Part model, mm, in its own coordinate system. Round coordinates to 2 decimals unless told otherwise and drop trailing zeros. Order: outer loops, then holes, each group sorted by start corner. A loop starts at its lowest first (then second) coordinate and runs counter-clockwise, first axis right, second up. Notation, with made-up numbers: (-12, -31.75) - (24, -31.75) arc R32 ccw to (24, 2.25) - close; hole circle Ø7 at (74, 56.5). An arc over 180 degrees is marked (long way). Answer as a JSON object with one key per item and string values.
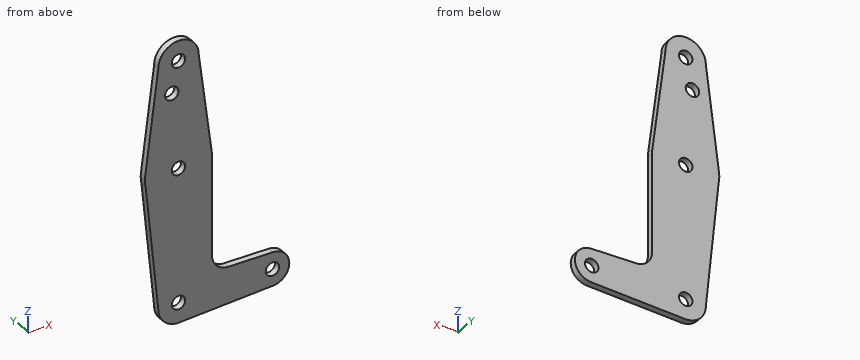
```python
from build123d import *

# Parameters (mm, degrees)
F0_R     = 3.175
F1_DEPTH = 3.048


with BuildPart() as f1:
    # F0 (on Front) → F1 (new body)
    with BuildSketch(Plane.XZ):
        with BuildLine():
            ThreePointArc((3.175, 0), (-2.2450640303, -2.2450640303), (0, 3.175))
            Line((0, 3.175), (0, 9.525))
            ThreePointArc((0, 9.525), (-6.7351920908, 6.7351920908), (-9.525, 0))
            ThreePointArc((-9.525, 0), (-6.7351920908, -6.7351920908), (0, -9.525))
            Line((0, -9.525), (0.6773435479, -9.500885786))
            ThreePointArc((0.6773435479, -9.500885786), (6.9705567315, -6.4912990883), (9.525, 0))
            Line((9.525, 0), (3.175, 0))
        make_face()
        with BuildLine():
            ThreePointArc((-9.525, 0), (-6.7351920908, 6.7351920908), (0, 9.525))
            Line((0, 9.525), (0, 47.625))
            ThreePointArc((0, 47.625), (-10.0526499203, 51.2134278751), (-15.5606435644, 60.3564356436))
            Line((-15.5606435644, 60.3564356436), (-9.525, 0))
        make_face()
        with BuildLine():
            Line((0, 47.625), (0, 9.525))
            ThreePointArc((0, 9.525), (6.7351920908, 6.7351920908), (9.525, 0))
            Line((9.525, 0), (36.5125, 0))
            ThreePointArc((36.5125, 0), (38.9239306999, 5.6979350945), (44.6930264481, 7.9337786959))
            Line((44.6930264481, 7.9337786959), (23.5817847096, 8.5804554297))
            ThreePointArc((23.5817847096, 8.5804554297), (18.1181482094, 10.9920171606), (15.875, 16.5269281715))
            Line((15.875, 16.5269281715), (15.875, 63.5))
            ThreePointArc((15.875, 63.5), (11.2253201513, 52.2746798487), (0, 47.625))
        make_face()
        with BuildLine():
            Line((36.5125, 0), (9.525, 0))
            ThreePointArc((9.525, 0), (6.9705567315, -6.4912990883), (0.6773435479, -9.500885786))
            Line((0.6773435479, -9.500885786), (44.7324052746, -7.9324746146))
            ThreePointArc((44.7324052746, -7.9324746146), (38.9380895153, -5.7116327839), (36.5125, 0))
        make_face()
        with BuildLine():
            ThreePointArc((-15.5606435644, 60.3564356436), (-10.0526499203, 51.2134278751), (0, 47.625))
            Line((0, 47.625), (0, 60.325))
            ThreePointArc((0, 60.325), (-3.175, 63.5), (0, 66.675))
            Line((0, 66.675), (0, 79.375))
            ThreePointArc((0, 79.375), (-10.4912828548, 75.4142187767), (-15.7474569047, 65.5082893304))
            ThreePointArc((-15.7474569047, 65.5082893304), (-15.8430821396, 64.5061676396), (-15.875, 63.5))
            Line((-15.875, 63.5), (-15.5606435644, 60.3564356436))
        make_face()
        with BuildLine():
            Line((0, 60.325), (0, 47.625))
            ThreePointArc((0, 47.625), (11.2253201513, 52.2746798487), (15.875, 63.5))
            ThreePointArc((15.875, 63.5), (15.8430821396, 64.5061676396), (15.7474569047, 65.5082893304))
            ThreePointArc((15.7474569047, 65.5082893304), (10.4912828548, 75.4142187767), (0, 79.375))
            Line((0, 79.375), (0, 66.675))
            ThreePointArc((0, 66.675), (2.2450640303, 65.7450640303), (3.175, 63.5))
            ThreePointArc((3.175, 63.5), (2.2450640303, 61.2549359697), (0, 60.325))
        make_face()
        with BuildLine():
            ThreePointArc((44.6930264481, 7.9337786959), (38.9239306999, 5.6979350945), (36.5125, 0))
            ThreePointArc((36.5125, 0), (38.9380895153, -5.7116327839), (44.7324052746, -7.9324746146))
            ThreePointArc((44.7324052746, -7.9324746146), (50.1616327839, -5.5119104847), (52.3875, 0))
            ThreePointArc((52.3875, 0), (50.1479350945, 5.5260693001), (44.6930264481, 7.9337786959))
        make_face()
        with BuildLine():
            ThreePointArc((47.625, 0), (44.45, -3.175), (41.275, 0))
            ThreePointArc((41.275, 0), (44.45, 3.175), (47.625, 0))
        make_face(mode=Mode.SUBTRACT)
        with BuildLine():
            ThreePointArc((0, -9.525), (0.3388863295, -9.5189695375), (0.6773435479, -9.500885786))
            Line((0.6773435479, -9.500885786), (0, -9.525))
        make_face()
        with BuildLine():
            ThreePointArc((-15.5652161214, 60.3791552277), (-15.5629339888, 60.3677946012), (-15.5606435644, 60.3564356436))
            Line((-15.5606435644, 60.3564356436), (-15.875, 63.5))
            Line((-15.875, 63.5), (-15.5652161214, 60.3791552277))
        make_face()
        with BuildLine():
            ThreePointArc((-15.875, 63.5), (-15.7973641936, 61.9319089516), (-15.5652161214, 60.3791552277))
            Line((-15.5652161214, 60.3791552277), (-15.875, 63.5))
        make_face()
        with BuildLine():
            ThreePointArc((0, 79.375), (10.4912828548, 75.4142187767), (15.7474569047, 65.5082893304))
            Line((15.7474569047, 65.5082893304), (9.525, 114.3))
            ThreePointArc((9.525, 114.3), (6.7351920908, 107.5648079092), (0, 104.775))
            Line((0, 104.775), (0, 100.0252))
            Line((0, 100.0252), (0, 79.375))
        make_face()
        with BuildLine():
            ThreePointArc((-15.7474569047, 65.5082893304), (-10.4912828548, 75.4142187767), (0, 79.375))
            Line((0, 79.375), (0, 100.0252))
            Line((0, 100.0252), (0, 104.775))
            ThreePointArc((0, 104.775), (-6.7351920908, 107.5648079092), (-9.525, 114.3))
            Line((-9.525, 114.3), (-15.7474569047, 65.5082893304))
        make_face()
        with Locations((-3.175, 100.0252)):
            Circle(F0_R, mode=Mode.SUBTRACT)
        with BuildLine():
            ThreePointArc((0, 104.775), (6.7351920908, 107.5648079092), (9.525, 114.3))
            ThreePointArc((9.525, 114.3), (0, 123.825), (-9.525, 114.3))
            ThreePointArc((-9.525, 114.3), (-6.7351920908, 107.5648079092), (0, 104.775))
        make_face()
        with BuildLine():
            ThreePointArc((3.175, 114.3), (2.2450640303, 112.0549359697), (0, 111.125))
            ThreePointArc((0, 111.125), (-2.2450640303, 116.5450640303), (3.175, 114.3))
        make_face(mode=Mode.SUBTRACT)
        with BuildLine():
            Line((0, 9.525), (0, 3.175))
            ThreePointArc((0, 3.175), (2.2450640303, 2.2450640303), (3.175, 0))
            Line((3.175, 0), (9.525, 0))
            ThreePointArc((9.525, 0), (6.7351920908, 6.7351920908), (0, 9.525))
        make_face()
    extrude(amount=F1_DEPTH)


solid = f1.part
```
Item 1: Cut at A-A (y = -1.8). State how many separate pieces and enclosed holes the cut face has, plus the area to 3 significant figures.
Taken from the geometry:
{"separate pieces": "1", "enclosed holes": "5", "area": "3,910 mm2"}
Item 2: Drop flat-ended pins along their axis: P1, Ø0.9, axis at y = -1, z = 51.5, coming from the +X side (3 decimals); P2, Ø10, axis at x = 0, z = 0, coming from the -Y side; P3, Ø5, axis at x = 0, z = 114.3, coming from the -Y side. Give the stop position or say it passes through.
Taken from the geometry:
{"P1": "x = 15.875", "P2": "y = -3.05", "P3": "through"}
Item 3: Cut at B-B (z = 20.5). Write the cut outline in (x, y) (3 decimals), plus the area to 3 significant figures.
Taken from the geometry:
{"outline": "(-11.575, -3.048) - (15.875, -3.048) - (15.875, 0) - (-11.575, 0) - close", "area": "83.7 mm2"}
Item 4: Probe L1, parallel to Z at x = 44.45, y = -1.1 (3 decimals); L2, parallel to Z at x = 0.5, y = -1.75; L3, parallel to Z at x = 1, y = -0.3. List the from-to ranges inside material, lowest first. Write a range as from..to.
Taken from the geometry:
{"L1": "-7.943..-3.175, 3.175..7.941", "L2": "-9.51..-3.14, 3.14..60.36, 66.64..111.16, 117.44..123.81", "L3": "-9.49..-3.01, 3.01..60.49, 66.51..111.29, 117.31..123.77"}
Item 5: Cut at C-C (x = 31). Write the cut outline in (y, z), plus the area to 3 significant figures.
Taken from the geometry:
{"outline": "(-3.05, -8.42) - (0, -8.42) - (0, 8.35) - (-3.05, 8.35) - close", "area": "51.1 mm2"}
